from build123d import *

# Parameters (mm, degrees)
SKETCH1_W           = 47
SKETCH1_H           = 30
SKETCH1_R           = 2.25
BOSS_EXTRUDE1_DEPTH = 3
SKETCH2_R           = 1.9
BOSS_EXTRUDE2_DEPTH = 43
CUT_EXTRUDE1_REACH  = 98.861
SKETCH3_R           = 3.5
CUT_EXTRUDE2_DEPTH  = 39


with BuildPart() as part:
    # Sketch1 → Boss-Extrude1 (new body)
    with BuildSketch(Plane.XY):
        with Locations((23.5, 15)):
            Rectangle(SKETCH1_W, SKETCH1_H)
        with Locations((16.5, 21)):
            Circle(SKETCH1_R, mode=Mode.SUBTRACT)
        with Locations((34.5, 21)):
            Circle(SKETCH1_R, mode=Mode.SUBTRACT)
    extrude(amount=BOSS_EXTRUDE1_DEPTH)

    # Sketch2 → Boss-Extrude2 (add)
    # profile 1 of 3: a face of its own
    with BuildSketch(Plane.ZY):
        Polygon((-75, 24.917096231), (-75, 3), (-61, 3), (-61, 33), align=None)
        with Locations(Location((-65.5, 16.5, 0), (0, 0, 270))):
            Circle(SKETCH2_R, mode=Mode.SUBTRACT)
    # profile 2 of 3: a face of its own
    with BuildSketch(Plane.ZY):
        Polygon((-75, 0), (0, 0), (0, 3), (-14, 3), (-61, 3), (-75, 3), align=None)
    # profile 3 of 3: a face of its own
    with BuildSketch(Plane.ZY):
        Polygon((-14, 3), (0, 3), (0, 30), (-14, 33), align=None)
        with Locations(Location((-9.5, 16.5, 0), (0, 0, 270))):
            Circle(SKETCH2_R, mode=Mode.SUBTRACT)
    extrude(amount=-BOSS_EXTRUDE2_DEPTH)

    # Cut-Extrude1: up to this face of the body (flat: up to its plane)
    cut_extrude1_end = Plane(part.part.faces().sort_by_distance((45, 15, 0))[0])
    # Sketch3 → Cut-Extrude1 (cut, up to the picked face)
    with BuildSketch(Plane(origin=(0, 0, -75), x_dir=(-1, 0, 0), z_dir=(0, 0, -1)), mode=Mode.PRIVATE) as cut_extrude1_sk1:
        with Locations((-34.5, 21)):
            Circle(SKETCH3_R)
    cut_extrude1_tool1 = split(extrude(cut_extrude1_sk1.sketch, amount=-CUT_EXTRUDE1_REACH, mode=Mode.PRIVATE), bisect_by=cut_extrude1_end, keep=Keep.BOTH, mode=Mode.PRIVATE)
    # Sketch3 → Cut-Extrude1 (cut, up to the picked face)
    with BuildSketch(Plane(origin=(0, 0, -75), x_dir=(-1, 0, 0), z_dir=(0, 0, -1)), mode=Mode.PRIVATE) as cut_extrude1_sk2:
        with Locations((-16.5, 21)):
            Circle(SKETCH3_R)
    cut_extrude1_tool2 = split(extrude(cut_extrude1_sk2.sketch, amount=-CUT_EXTRUDE1_REACH, mode=Mode.PRIVATE), bisect_by=cut_extrude1_end, keep=Keep.BOTH, mode=Mode.PRIVATE)
    add(cut_extrude1_tool1.solids().sort_by(Axis((34.5, 21, -75), (0, 0, 1)))[0], mode=Mode.SUBTRACT)
    add(cut_extrude1_tool2.solids().sort_by(Axis((16.5, 21, -75), (0, 0, 1)))[0], mode=Mode.SUBTRACT)

    # Sketch4 → Cut-Extrude2 (cut)
    with BuildSketch(Plane(origin=(43, 0, 0), x_dir=(0, 0, -1), z_dir=(1, 0, 0))):
        Polygon((9.5, 13.209103466), (12.35, 14.854551733), (12.35, 18.145448267), (9.5, 19.790896534), (6.65, 18.145448267), (6.65, 14.854551733), align=None)
        Polygon((65.5, 13.209103466), (68.35, 14.854551733), (68.35, 18.145448267), (65.5, 19.790896534), (62.65, 18.145448267), (62.65, 14.854551733), align=None)
    extrude(amount=-CUT_EXTRUDE2_DEPTH, mode=Mode.SUBTRACT)


solid = part.part
Here's how the part is built. I have some questions about the finished solid (model axes, mm). A direction names the side the tool comes from. Give positions to 0.01 mm unless a question says otherwise; leave off trailing zeros. Loops run counter-clockwise (first coordinate to the right, second up) from the corner with the lowest first, then second, coordinate; pieces in that order, holes last. Notation, with made-up numbers: (45, 84.25) -> (103, 84.25) arc R17 cw to (103, 99.25) -> close; hole circle Ø6 at (17, 2.25). An arc over 180 degrees is marked (long way). One line per item, written item: value.
Q1. Suppose I cut it at A-A on y = 16.5. Please give me the cut outline in (x, z), then the cut area to 3 significant figures.
Answers follow:
outline: (0, -75) -> (43, -75) -> (43, -68.35) -> (4, -68.35) -> (4, -67.4) -> (0, -67.4) -> close; (0, -63.6) -> (4, -63.6) -> (4, -62.65) -> (43, -62.65) -> (43, -61) -> (0, -61) -> close; (0, -14) -> (43, -14) -> (43, -12.35) -> (4, -12.35) -> (4, -11.4) -> (0, -11.4) -> close; (0, -7.6) -> (4, -7.6) -> (4, -6.65) -> (43, -6.65) -> (43, 0) -> (47, 0) -> (47, 3) -> (0, 3) -> close
area: 870 mm^2
Q2. I'm going to push flat-ended pins straight in: pin 1 Ø6.5 at (y, z) = (16, -9.5) entering from +X; pin 2 Ø4.5 at (x, y) = (45.5, 15) entering from -Z; pin 3 Ø3.5 at (x, z) = (35, 1.5) entering from +Y. Where does each tip first touch, or does it pass through?
Answers follow:
pin 1: x = 43
pin 2: z = 0
pin 3: y = 30.05
Q3. If I drill on line 1 along Z through (x, y) = (1.95, 16.5); line 2 along Z through (x, y) = (14.5, 17.5); line 3 along Z through (x, y) = (28, 11.5), over which ranges is the centre line in solid material (lowest first)?
Answers follow:
line 1: -75 to -67.4, -63.6 to -61, -14 to -11.4, -7.6 to 3
line 2: -75 to -68.35, -62.65 to -61, -14 to -12.35, -6.65 to 3
line 3: -75 to -61, -14 to 3
Q4. On a 3-axis mill with a long thin cutter (end or side, diameter ignored), from which of +Z, -Z, +X, -X, +Y, -Y can I reach the whole of each face in a straight line? I mean faces 1 (the face through (37, 21, 0)), 2 (the face through (17.538, 19.004, 1.479)), 3 (the face through (21, 18, -61)), 4 (the face through (25.598, 18.98, -8.095)). Say none if no direction works.
Answers follow:
face 1: -Z
face 2: +Z, -Z
face 3: +X, -X, +Y
face 4: +X
Q5. Suppose I cut it at B-B on x = 9. Please give me the cut outline in (y, z), then the cut area to 3 significant figures.
Answers follow:
outline: (0, -75) -> (24.92, -75) -> (33, -61) -> (3, -61) -> (3, -14) -> (33, -14) -> (30, 0) -> (30, 3) -> (0, 3) -> close; hole (13.21, -65.5) -> (14.85, -68.35) -> (18.15, -68.35) -> (19.79, -65.5) -> (18.15, -62.65) -> (14.85, -62.65) -> close; hole (13.21, -9.5) -> (14.85, -12.35) -> (18.15, -12.35) -> (19.79, -9.5) -> (18.15, -6.65) -> (14.85, -6.65) -> close
area: 1,020 mm^2
Q6. Suppose I cut it at C-C on y = 21. State how many separate pieces and enclosed holes the cut face has, then the cut area to 3 significant figures.
Answers follow:
separate pieces: 6
enclosed holes: 0
area: 926 mm^2
Q7. We'd pull the mould along Y, two halves only. Please class faces 5 (the face through (23, 0, -37)), 6 (the face through (4, 15, -64)), 7 (the face through (21, 18, -14)): pulls with the +Y half, pulls with the -Y half, needs draft (parallel to the pull), parting line crosses it, or undercut.
Answers follow:
face 5: pulls with the -Y half
face 6: undercut
face 7: needs draft
Q8. Suppose I cut it at D-D on z = -10.5. Please give me the cut outline in (x, y).
Answers follow:
outline: (0, 0) -> (43, 0) -> (43, 13.79) -> (4, 13.79) -> (4, 14.88) -> (0, 14.88) -> close; (0, 18.12) -> (4, 18.12) -> (4, 19.21) -> (13.49, 19.21) arc R3.5 cw (long way) to (19.51, 19.21) -> (31.49, 19.21) arc R3.5 cw (long way) to (37.51, 19.21) -> (43, 19.21) -> (43, 32.25) -> (0, 32.25) -> close
